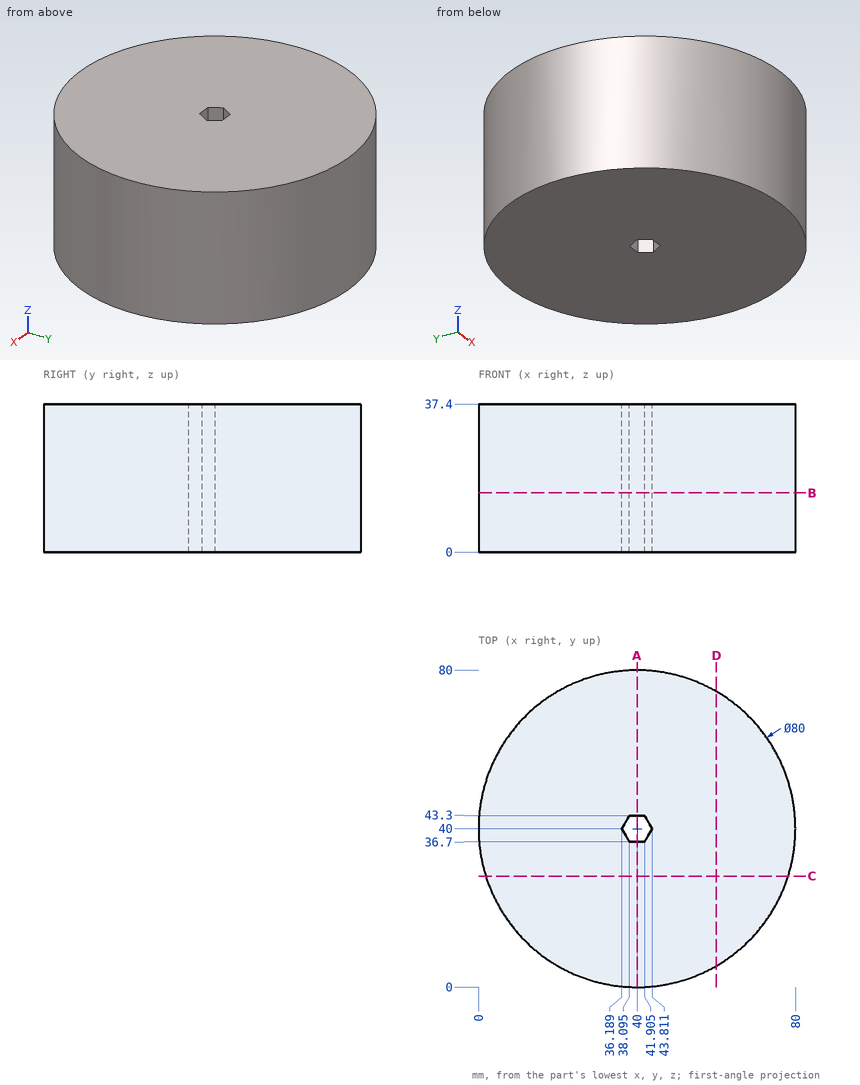
Job drawing, mm, ordinate dimensions from the low corner. One solid piece. Round coordinates to 2 decimals unless told otherwise and drop trailing zeros. Loops run counter-clockwise (first coordinate to the right, second up) from the corner with the lowest first, then second, coordinate; pieces in that order, holes last.
Item 1: Cut at A-A, the plane x = 40. Give the cut face in (y, z).
Item 2: Cut at C-C, the plane y = 28. Give the cut face in (x, z).
Item 3: Cut at D-D, the plane x = 60. Give the cut face in (y, z).
Item 4: Cut at B-B, the plane z = 15. Give the cut face in (x, y) (1 decimal), then the cut area to 3 significant figures.
Item 5: Drill centre lines: line 1 (X direction, y = 37, z = 35.5); line 2 (X direction, y = 72, z = 6.5); line 3 (X direction, y = 68.5, z = 13.5) (1 decimal). Where is each one in solid material? Low to high.
Item 6: Drop flat-ended pins along their axis: P1, Ø6, axis at x = 27.5, z = 15, coming from the +Y side (1 decimal); P2, Ø2, axis at y = 12.5, z = 24, coming from the -X side; P3, Ø1.5, axis at x = 54.5, z = 7, coming from the -Y side. Give the stop position or say it passes through.
A:
1. outline: (0, 0) - (36.7, 0) - (36.7, 37.4) - (0, 37.4) - close; (43.3, 0) - (80, 0) - (80, 37.4) - (43.3, 37.4) - close
2. outline: (1.84, 0) - (78.16, 0) - (78.16, 37.4) - (1.84, 37.4) - close
3. outline: (5.36, 0) - (74.64, 0) - (74.64, 37.4) - (5.36, 37.4) - close
4. outline: circle Ø80 at (40, 40); hole (36.2, 40) - (38.1, 36.7) - (41.9, 36.7) - (43.8, 40) - (41.9, 43.3) - (38.1, 43.3) - close
4. area: 4,990 mm2
5. line 1: x = 0.11 to 37.92, 42.08 to 79.89
5. line 2: x = 16 to 64
5. line 3: x = 11.9 to 68.1
6. P1: stops at y = 78.9
6. P2: stops at x = 10.04
6. P3: stops at y = 2.44
